from build123d import *

# Parameters (mm, degrees)
BOSS_EXTRUDE1_DEPTH = 6.5
BOSS_EXTRUDE2_DEPTH = 3
BOSS_EXTRUDE3_DEPTH = 3
SKETCH10_W          = 9.5
SKETCH10_H          = 5
BOSS_EXTRUDE4_DEPTH = 15.78
SKETCH11_W          = 9.5
SKETCH11_H          = 2
BOSS_EXTRUDE5_DEPTH = 40
BOSS_EXTRUDE6_DEPTH = 6.09393
SKETCH14_R          = 1.8
CUT_EXTRUDE1_DEPTH  = 6.3
SKETCH15_W          = 51.153217575
SKETCH15_H          = 21.210560201
CUT_EXTRUDE3_DEPTH  = 19.78
SKETCH18_W          = 3
SKETCH18_H          = 3
BOSS_EXTRUDE7_DEPTH = 6.5
FILLET1_R           = 0.75
BOSS_EXTRUDE8_DEPTH = 1.5
FILLET2_R           = 0.75
BOSS_EXTRUDE9_DEPTH = 10


with BuildPart() as part:
    # Sketch3 → Revolve1 (revolve)
    with BuildSketch(Plane.XY):
        Polygon((-62.694264441, 11.733728816), (-64.884531744, 11.733728816), (-64.884531744, 5.639799249), (-60.884531744, 5.639799249), (-60.884531744, 6.650679103), (-62.884531744, 6.650679103), (-62.884531744, 10.250679103), (-60.884531744, 10.250679103), (-60.884531744, 11.733728816), align=None)
    revolve(axis=Axis((-49.744264441, 0, 0), (0, 1, 0)))

    # Sketch7 → Boss-Extrude1 (add)
    with BuildSketch(Plane(origin=(0, 11.733728816, 0), x_dir=(1, 0, 0), z_dir=(0, 1, 0))):
        with BuildLine():
            Line((-50.244264441, 15.132008921), (-50.244264441, 13.130751112))
            ThreePointArc((-50.244264441, 13.130751112), (-49.744264441, 13.140267302), (-49.244264441, 13.130751112))
            Line((-49.244264441, 13.130751112), (-49.244264441, 15.132008921))
            ThreePointArc((-49.244264441, 15.132008921), (-49.744264441, 15.140267302), (-50.244264441, 15.132008921))
        make_face()
    extrude(amount=BOSS_EXTRUDE1_DEPTH)

    # Sketch8 → Boss-Extrude2 (add)
    with BuildSketch(Plane(origin=(0, 18.233728816, 0), x_dir=(1, 0, 0), z_dir=(0, 1, 0))):
        with BuildLine():
            Line((-50.244264441, 15.132008921), (-50.244264441, 13.130751112))
            Line((-50.244264441, 13.130751112), (-50.244264441, -6.369248888))
            Line((-50.244264441, -6.369248888), (-49.244264441, -6.369248888))
            Line((-49.244264441, -6.369248888), (-49.244264441, 13.130751112))
            Line((-49.244264441, 13.130751112), (-49.244264441, 15.132008921))
            ThreePointArc((-49.244264441, 15.132008921), (-49.744264441, 15.140267302), (-50.244264441, 15.132008921))
        make_face()
    extrude(amount=-BOSS_EXTRUDE2_DEPTH)

    # Sketch9 → Boss-Extrude3 (add)
    with BuildSketch(Plane(origin=(0, 11.733728816, 0), x_dir=(1, 0, 0), z_dir=(0, 1, 0))):
        with BuildLine():
            Line((-54.494264441, 14.375854548), (-54.494264441, 39.375854548))
            Line((-54.494264441, 39.375854548), (-44.994264441, 39.375854548))
            Line((-44.994264441, 39.375854548), (-44.994264441, 14.375854548))
            ThreePointArc((-44.994264441, 14.375854548), (-47.092177082, 14.906177465), (-49.244264441, 15.132008921))
            ThreePointArc((-49.244264441, 15.132008921), (-49.744264441, 15.140267302), (-50.244264441, 15.132008921))
            ThreePointArc((-50.244264441, 15.132008921), (-52.3963518, 14.906177465), (-54.494264441, 14.375854548))
        make_face()
    extrude(amount=-BOSS_EXTRUDE3_DEPTH)

    # Sketch10 → Boss-Extrude4 (add)
    with BuildSketch(Plane.XZ.offset(-8.733728816)):
        with Locations((-49.744264441, -36.875854548)):
            Rectangle(SKETCH10_W, SKETCH10_H)
    extrude(amount=BOSS_EXTRUDE4_DEPTH)

    # Sketch11 → Boss-Extrude5 (add)
    with BuildSketch(Plane(origin=(0, 0, -39.375854548), x_dir=(-1, 0, 0), z_dir=(0, 0, -1))):
        with Locations((49.744264441, -6.046271184)):
            Rectangle(SKETCH11_W, SKETCH11_H)
    extrude(amount=BOSS_EXTRUDE5_DEPTH)

    # Sketch13 → Boss-Extrude6 (add)
    with BuildSketch(Plane(origin=(0, 11.733728816, 0), x_dir=(1, 0, 0), z_dir=(0, 1, 0))):
        with BuildLine():
            Line((-28.603997139, 3.15), (-34.935307895, 3.15))
            ThreePointArc((-34.935307895, 3.15), (-34.603997139, 0), (-34.935307895, -3.15))
            Line((-34.935307895, -3.15), (-28.603997139, -3.15))
            Line((-28.603997139, -3.15), (-28.603997139, 3.15))
        make_face()
        with BuildLine():
            Line((-70.884531744, 3.15), (-70.884531744, -3.15))
            Line((-70.884531744, -3.15), (-64.553220987, -3.15))
            ThreePointArc((-64.553220987, -3.15), (-64.884531744, 0), (-64.553220987, 3.15))
            Line((-64.553220987, 3.15), (-70.884531744, 3.15))
        make_face()
    extrude(amount=-BOSS_EXTRUDE6_DEPTH)

    # Sketch14 → Cut-Extrude1 (cut)
    with BuildSketch(Plane.XY.offset(3.15)):
        with Locations((-31.769652517, 8.686764033)):
            Circle(SKETCH14_R)
        with Locations((-67.718876365, 8.686764033)):
            Circle(SKETCH14_R)
    extrude(amount=-CUT_EXTRUDE1_DEPTH, mode=Mode.SUBTRACT)

    # Sketch15 → Cut-Extrude3 (cut, through all)
    with BuildSketch(Plane(origin=(0, 11.733728816, 0), x_dir=(1, 0, 0), z_dir=(0, 1, 0))):
        with Locations((-49.018725857, -10.6052801)):
            Rectangle(SKETCH15_W, SKETCH15_H)
    extrude(amount=-CUT_EXTRUDE3_DEPTH, mode=Mode.SUBTRACT)

    # Sketch18 → Boss-Extrude7 (add)
    with BuildSketch(Plane(origin=(0, 11.733728816, 0), x_dir=(1, 0, 0), z_dir=(0, 1, 0))):
        with Locations((-49.744264441, 13.632008921)):
            Rectangle(SKETCH18_W, SKETCH18_H)
    extrude(amount=BOSS_EXTRUDE7_DEPTH)

    # Fillet1
    fillet1_edges = [part.edges().sort_by_distance(p)[0] for p in [
        (-50.744264441, 11.733728816, -15.132008921),
        (-48.744264441, 11.733728816, -15.132008921),
        (-49.744264441, 11.733728816, -12.132008921),
        (-48.244264441, 11.733728816, -13.632008921),
        (-51.244264441, 11.733728816, -13.632008921),
        (-49.744264441, 11.733728816, -15.140267302),
    ]]
    fillet(fillet1_edges, radius=FILLET1_R)

    # Sketch19 → Boss-Extrude8 (add)
    with BuildSketch(Plane(origin=(0, 18.233728816, 0), x_dir=(1, 0, 0), z_dir=(0, 1, 0))):
        with BuildLine():
            Line((-50.244264441, 15.132008921), (-51.244264441, 15.132008921))
            Line((-51.244264441, 15.132008921), (-51.244264441, 12.132008921))
            Line((-51.244264441, 12.132008921), (-50.244264441, 12.132008921))
            Line((-50.244264441, 12.132008921), (-50.244264441, -6.369248888))
            Line((-50.244264441, -6.369248888), (-49.244264441, -6.369248888))
            Line((-49.244264441, -6.369248888), (-49.244264441, 12.132008921))
            Line((-49.244264441, 12.132008921), (-48.244264441, 12.132008921))
            Line((-48.244264441, 12.132008921), (-48.244264441, 15.132008921))
            Line((-48.244264441, 15.132008921), (-49.244264441, 15.132008921))
            ThreePointArc((-49.244264441, 15.132008921), (-49.744264441, 15.140267302), (-50.244264441, 15.132008921))
        make_face()
    extrude(amount=BOSS_EXTRUDE8_DEPTH)

    # Fillet2
    fillet2_edges = [part.edges().sort_by_distance(p)[0] for p in [
        (-50.244264441, 17.483728816, -12.132008921),
        (-49.244264441, 17.483728816, -12.132008921),
    ]]
    fillet(fillet2_edges, radius=FILLET2_R)

    # Sketch20 → Boss-Extrude9 (add)
    with BuildSketch(Plane(origin=(0, 0, -79.375854548), x_dir=(-1, 0, 0), z_dir=(0, 0, -1))):
        with BuildLine():
            Line((37.244264441, -20.046271184), (39.244264441, -20.046271184))
            add(Edge.make_bspline(
                [(39.244264441, -20.046271184), (39.582311707, -9.650122804), (44.994264441, -7.046271184)],
                knots=[0, 0, 0, 0.599407443, 0.599407443, 0.599407443], degree=2))
            Line((44.994264441, -7.046271184), (54.494264441, -7.046271184))
            add(Edge.make_bspline(
                [(54.494264441, -7.046271184), (59.906217176, -9.650122804), (60.244264441, -20.046271184)],
                knots=[0.400592557, 0.400592557, 0.400592557, 1, 1, 1], degree=2))
            Line((60.244264441, -20.046271184), (62.244264441, -20.046271184))
            add(Edge.make_bspline(
                [(62.244264441, -20.046271184), (61.29176104, -7.746792571), (54.494264441, -5.046271184)],
                knots=[0, 0, 0, 0.639930482, 0.639930482, 0.639930482], degree=2))
            Line((54.494264441, -5.046271184), (44.994264441, -5.046271184))
            add(Edge.make_bspline(
                [(37.244264441, -20.046271184), (38.196767843, -7.746792571), (44.994264441, -5.046271184)],
                knots=[0, 0, 0, 0.639930482, 0.639930482, 0.639930482], degree=2))
        make_face()
    extrude(amount=-BOSS_EXTRUDE9_DEPTH)


solid = part.part
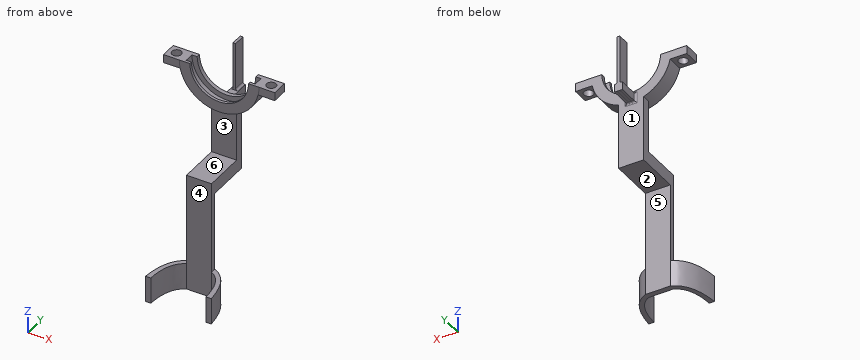
Can you work these out from the model? Positions are in its coordinate system, mm. Face numbers are marked on the shaded views. A direction names the side the tool comes from. Give positions to 0.01 mm unless a question says otherwise; leave off trailing zeros. Order: outer loops, then holes, each group sorted by start corner. A loop starts at its lowest first (then second) coordinate and runs counter-clockwise, first axis right, second up. Notation, with made-up numbers: M 42,34.5 L 91,34.5 A22 ccw 91,51.5 Z; hole C 66,6 d6. An arc over 180 degrees is marked long. Use a Markdown table: item, result. Add a question column.
Item 1: Suppose I cut it at A-A (z = -7.5). List the corners of the cut face in (x, y) for me, then the cut area to 3 significant figures.
Item 2: Suppose I cut it at B-B (y = 14). List the corners of the cut face in (x, z) for me, then the cut area to 3 significant figures.
Item 3: If I drill on L1, parallel to Y at x = -46.5, z = -54.5; L2, parallel to X at y = 17, z = -15; L3, parallel to X at y = -7, z = -58.5, over which ranges is the centre line in solid material (lowest first)? Write a range as [from, to].
Item 4: Suppose I cut it at C-C (z = -67). List the corners of the cut face in (x, y) for me.
Item 5: We'd pull the mould along Z, two halves only. Please class the marked faces 1, 2 and 3: +Z half, -Z half, draft (parallel to the pull), parting line (faces both ways), or undercut.
Item 6: Will these pins go through, and if not, where does the flat tip stop? pin 1 (12 mm diameter, centred on x = -42, z = -41, fed in from -Y); pin 2 (4 mm diameter, centred on x = -54, z = -4.5, fed in from +Y); pin 3 (6 mm diameter, centred on x = -41.5, y = -16, fed in from +Z); pin 4 (3.5 mm diameter, centred on y = 16.5, z = -13.5, fed in from -X).
Item 7: Suppose I cut it at D-D (y = -1). List the corners of the cut face in (x, z) for me.
Item 8: For the marked faces 4, 5 and 6, which set-ups out of +Z, -Z, +X, -X, +Y, -Y let a thin tool reach every point of the face, with its end or its side?
Answer sheet:
| question | item | result |
|---|---|---|
| 1 | outline | M -62.9,5.64 L -57.98,5.64 L -57.98,6.65 L -60.53,6.65 L -60.53,10.25 L -57.98,10.25 L -57.98,11.73 L -62.9,11.73 Z; M -50.24,15.23 L -49.24,15.23 L -49.24,19.73 L -50.24,19.73 Z; M -41.51,5.64 L -36.59,5.64 L -36.59,11.73 L -41.51,11.73 L -41.51,10.25 L -38.95,10.25 L -38.95,6.65 L -41.51,6.65 Z |
| 1 | area | 46.0 mm² |
| 2 | outline | M -51.24,-15.13 L -50.24,-15.13 A15.14 ccw -49.24,-15.13 L -48.24,-15.13 L -48.24,-12.13 L -51.24,-12.13 Z |
| 2 | area | 9.01 mm² |
| 3 | L1 | y = [-7.05, -5.05] |
| 3 | L2 | x = [-51.24, -48.24] |
| 3 | L3 | x = [-54.49, -44.99] |
| 4 | outline | M -54.49,-7.05 L -44.99,-7.05 L -44.99,-5.05 L -54.49,-5.05 Z |
| 5 | face 1 | draft |
| 5 | face 2 | -Z half |
| 5 | face 3 | undercut |
| 6 | pin 1 | stops at y = -7.05 |
| 6 | pin 2 | passes through |
| 6 | pin 3 | stops at z = -69.38 |
| 6 | pin 4 | stops at x = -51.24 |
| 7 | outline | M -54.49,-39.38 L -44.99,-39.38 L -44.99,-34.38 L -54.49,-34.38 Z |
| 8 | face 4 | +Z, -Z, -Y |
| 8 | face 5 | -Z, +X, -X, +Y |
| 8 | face 6 | +X, -X, -Y |
